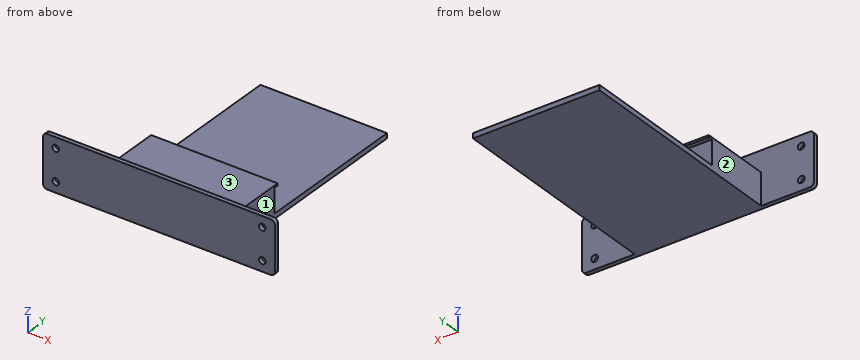
from build123d import *

# Parameters (mm, degrees)
SKETCH_1_W          = 110
SKETCH_1_H          = 25
SKETCH_1_R          = 1.6
EXTRUDE_1_DEPTH     = 2
SKETCH_2_W          = 60
SKETCH_2_H          = 15
EXTRUDE_2_DEPTH     = 113
CUT_EXTRUDE_1_DEPTH = 60
FILLET_1_R          = 2
FILLET_2_R          = 2
FILLET_3_R          = 2
FILLET_4_R          = 2
CUT_EXTRUDE_3_DEPTH = 144.5487722
SKETCH_8_W          = 60
SKETCH_8_H          = 6
CUT_EXTRUDE_4_DEPTH = 128.690093586


with BuildPart() as part:
    # 草图1 → 凸台-拉伸1 (new body)
    with BuildSketch(Plane(origin=(0, 0, 0), x_dir=(1, 0, 0), z_dir=(0, 1, 0))):
        Rectangle(SKETCH_1_W, SKETCH_1_H)
        with Locations(Location((-49, 7.5, 0), (0, 0, 270))):
            Circle(SKETCH_1_R, mode=Mode.SUBTRACT)
        with Locations(Location((49, 7.5, 0), (0, 0, 90))):
            Circle(SKETCH_1_R, mode=Mode.SUBTRACT)
        with Locations(Location((49, -7.5, 0), (0, 0, 270))):
            Circle(SKETCH_1_R, mode=Mode.SUBTRACT)
        with Locations(Location((-49, -7.5, 0), (0, 0, 90))):
            Circle(SKETCH_1_R, mode=Mode.SUBTRACT)
    extrude(amount=EXTRUDE_1_DEPTH)

    # 草图2 → 凸台-拉伸2 (add)
    with BuildSketch(Plane(origin=(0, 115, 0), x_dir=(1, 0, 0), z_dir=(0, 1, 0))):
        with Locations((0, 5)):
            Rectangle(SKETCH_2_W, SKETCH_2_H)
    extrude(amount=-EXTRUDE_2_DEPTH)

    # 草图3 → 切除-拉伸1 (cut)
    with BuildSketch(Plane(origin=(30, 0, 0), x_dir=(0, 0, -1), z_dir=(1, 0, 0))):
        Polygon((-2.5, 36), (-1.5, 36), (-1.5, 34), (10.1, 34), (10.1, 113), (-1.5, 113), (-1.5, 111), (-2.5, 111), align=None)
    extrude(amount=-CUT_EXTRUDE_1_DEPTH, mode=Mode.SUBTRACT)

    # 圆角1
    fillet_1_edges = [part.edges().sort_by_distance(p)[0] for p in [
        (55, 1, 12.5),
    ]]
    fillet(fillet_1_edges, radius=FILLET_1_R)

    # 圆角2
    fillet_2_edges = [part.edges().sort_by_distance(p)[0] for p in [
        (55, 1, -12.5),
    ]]
    fillet(fillet_2_edges, radius=FILLET_2_R)

    # 圆角3
    fillet_3_edges = [part.edges().sort_by_distance(p)[0] for p in [
        (-55, 1, -12.5),
    ]]
    fillet(fillet_3_edges, radius=FILLET_3_R)

    # 圆角4
    fillet_4_edges = [part.edges().sort_by_distance(p)[0] for p in [
        (-55, 1, 12.5),
    ]]
    fillet(fillet_4_edges, radius=FILLET_4_R)

    # 草图7 → 切除-拉伸3 (cut, through all)
    with BuildSketch(Plane(origin=(30, 0, 0), x_dir=(0, 0, -1), z_dir=(1, 0, 0))):
        Polygon((10.125373214, 107), (10.1, 113), (-1.5, 113), (-1.5, 110), (-2.572411073, 110), (-2.572411073, 115), (12.5, 115), (12.5, 107), align=None)
    extrude(amount=-CUT_EXTRUDE_3_DEPTH, mode=Mode.SUBTRACT)

    # 草图8 → 切除-拉伸4 (cut, through all)
    with BuildSketch(Plane.XY.offset(-10.1)):
        with Locations((0, 110)):
            Rectangle(SKETCH_8_W, SKETCH_8_H)
    extrude(amount=-CUT_EXTRUDE_4_DEPTH, mode=Mode.SUBTRACT)


solid = part.part
Could you check a few things on this model? Use its own coordinates, in mm. Face numbers are marked on the shaded views. A direction names the side the tool comes from. Round coordinates to 2 decimals unless told otherwise and drop trailing zeros. Loops run counter-clockwise (first coordinate to the right, second up) from the corner with the lowest first, then second, coordinate; pieces in that order, holes last. Notation, with made-up numbers: (-31, 42) - (-4, 42) arc R19 ccw to (-4, 57) - close; hole circle Ø1 at (-36, -13). An arc over 180 degrees is marked (long way). Write item = value, one per line.
1) On a 3-axis mill with a long thin cutter (end or side, diameter ignored), from which of +Z, -Z, +X, -X, +Y, -Y can I reach the whole of each face in a straight line? I mean the marked faces 1, 2 and 3. Say none if no direction works.
Computed:
face_1 = +Z, -Z, +X, +Y
face_2 = +Z, -Z, -X, +Y
face_3 = +Z, +X, -X, +Y
2) Imagine slicing it at D-D (x = 22.5). Please give me the cut outline in (y, z).
Computed:
outline = (0, -12.5) - (107, -12.5) - (107, -10.1) - (34, -10.1) - (34, 1.5) - (36, 1.5) - (36, 2.5) - (2, 2.5) - (2, 12.5) - (0, 12.5) - close
3) I'm going to push flat-ended pins straight in: P1, Ø10, axis at y = 85, z = -8, coming from the -X side; P2, Ø6, axis at y = 29.5, z = 4, coming from the +X side; P3, Ø6, axis at x = -43.5, z = -4.5, coming from the +Y side. Where does each tip first touch, or does it pass through?
Computed:
P1 = -30
P2 = 30
P3 = 2
4) Imagine slicing it at A-A (z = 7.5). Please give me the cut outline in (x, y).
Computed:
outline = (-55, 0) - (-50.6, 0) - (-50.6, 2) - (-55, 2) - close; (-47.4, 0) - (47.4, 0) - (47.4, 2) - (-47.4, 2) - close; (50.6, 0) - (55, 0) - (55, 2) - (50.6, 2) - close
5) Imagine slicing it at C-C (z = -7.5). Please give me the cut outline in (x, y), and give its area (3 significant figures).
Computed:
outline = (-55, 0) - (-50.6, 0) - (-50.6, 2) - (-55, 2) - close; (-47.4, 0) - (47.4, 0) - (47.4, 2) - (30, 2) - (30, 34) - (-30, 34) - (-30, 2) - (-47.4, 2) - close; (50.6, 0) - (55, 0) - (55, 2) - (50.6, 2) - close
area = 2,130 mm2
6) I need wall thicknesses on line 1 along X through (y, z) = (0.55, -7.5); line 2 along Y through (x, z) = (-47, -4.5); line 3 along Y through (x, z) = (13, -6). Which ranges of each line are inside material? Lowest first, please. Write a range as from..to.
Computed:
line_1 = -55..-50.6, -47.4..47.4, 50.6..55
line_2 = 0..2
line_3 = 0..34
7) Imagine slicing it at B-B (x = -49). Please give me the cut outline in (y, z), and give its area (3 significant figures).
Computed:
outline = (0, -12.5) - (2, -12.5) - (2, -9.1) - (0, -9.1) - close; (0, -5.9) - (2, -5.9) - (2, 5.9) - (0, 5.9) - close; (0, 9.1) - (2, 9.1) - (2, 12.5) - (0, 12.5) - close
area = 37.2 mm2
